from build123d import *

# Parameters (mm, degrees)
SKETCH1_W           = 863.6
SKETCH1_H           = 88.9
BOSS_EXTRUDE1_DEPTH = 38.1
SKETCH3_W           = 88.9
SKETCH3_H           = 38.1
CUT_EXTRUDE2_DEPTH  = 39.1
SKETCH2_W           = 88.9
SKETCH2_H           = 38.1
CUT_EXTRUDE3_DEPTH  = 39.1
SKETCH4_W           = 69.85
SKETCH4_H           = 18.945503639
CUT_EXTRUDE4_DEPTH  = 89.9


with BuildPart() as part:
    # Sketch1 → Boss-Extrude1 (new body)
    with BuildSketch(Plane(origin=(0, 0, 0), x_dir=(1, 0, 0), z_dir=(0, 1, 0))):
        with Locations((431.8, 44.45)):
            Rectangle(SKETCH1_W, SKETCH1_H)
    extrude(amount=BOSS_EXTRUDE1_DEPTH)

    # Sketch3 → Cut-Extrude2 (cut, through all)
    with BuildSketch(Plane(origin=(0, 38.1, 0), x_dir=(1, 0, 0), z_dir=(0, 1, 0))):
        with Locations((44.45, 19.05)):
            Rectangle(SKETCH3_W, SKETCH3_H)
    extrude(amount=-CUT_EXTRUDE2_DEPTH, mode=Mode.SUBTRACT)

    # Sketch2 → Cut-Extrude3 (cut, through all)
    with BuildSketch(Plane.XZ):
        with Locations((819.15, -69.85)):
            Rectangle(SKETCH2_W, SKETCH2_H)
    extrude(amount=-CUT_EXTRUDE3_DEPTH, mode=Mode.SUBTRACT)

    # Sketch4 → Cut-Extrude4 (cut, through all)
    with BuildSketch(Plane(origin=(0, 0, -88.9), x_dir=(-1, 0, 0), z_dir=(0, 0, -1))):
        with Locations((-490.648634291, 28.627248181)):
            Rectangle(SKETCH4_W, SKETCH4_H)
    extrude(amount=-CUT_EXTRUDE4_DEPTH, mode=Mode.SUBTRACT)


solid = part.part
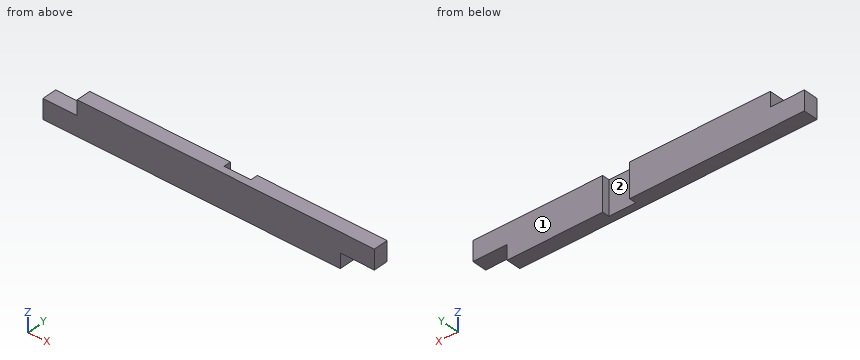
Part model, mm, in its own coordinate system. Face numbers are marked on the shaded views. Coordinates: 2 decimals unless noted, no trailing zeros. Write each loop counter-clockwise with the first axis right and the second up, starting at its lowest first coordinate (ties: lowest second). Pieces come first, ordered by that corner, then holes. Notation, with made-up numbers: M 54.5,-17 L 108.5,-17 A30 ccw 108.5,20 Z; hole C 21.25,-11 d11. An arc over 180 degrees is marked long. Return JSON: item names as keys, results as strings.
1. Saw through at A-A, the plane y = 29.5. Write the cut outline in (x, z), then the cut area to 3 significant figures.
Determined:
{"outline": "M 0,-88.9 L 455.72,-88.9 L 455.72,0 L 88.9,0 L 88.9,-38.1 L 0,-38.1 Z; M 525.57,-88.9 L 774.7,-88.9 L 774.7,-50.8 L 863.6,-50.8 L 863.6,0 L 525.57,0 Z", "area": "63,800 mm²"}
2. Probe L1, parallel to X at y = 32.5, z = -26; L2, parallel to X at y = 19.5, z = -59.5; L3, parallel to X at y = 8, z = -22.5. List the from-to ranges inside material, lowest first.
Determined:
{"L1": "88.9 to 455.72, 525.57 to 863.6", "L2": "0 to 455.72, 525.57 to 774.7", "L3": "88.9 to 863.6"}
3. Flat gauge pins, fed straight in: pin 1 Ø2 at (y, z) = (11, -69) entering from +X; pin 2 Ø2 at (x, y) = (317, 20.5) entering from +Z; pin 3 Ø1.5 at (y, z) = (8, -37) entering from -X; pin 4 Ø19 at (x, y) = (812, 24.5) entering from -Z. Where does each tip first touch, or does it go through?
Determined:
{"pin 1": "x = 774.7", "pin 2": "z = 0", "pin 3": "x = 88.9", "pin 4": "z = -50.8"}
4. Pull direction X, two halves, no side cores. Call the marked faces 1 and 2: pulls with the +X half, pulls with the -X half, needs draft (parallel to the pull), parting line crosses it, or undercut.
Determined:
{"face 1": "needs draft", "face 2": "undercut"}
5. Saw through at B-B, the plane z = -70.5. Write the cut outline in (x, y).
Determined:
{"outline": "M 0,0 L 774.7,0 L 774.7,38.1 L 525.57,38.1 L 525.57,19.15 L 455.72,19.15 L 455.72,38.1 L 0,38.1 Z"}
